from build123d import *

# Parameters (mm, degrees)
SKETCH_2_W               = 120
SKETCH_2_H               = 66
SKETCH_2_W_2             = 112
SKETCH_2_H_2             = 58
EXTRUDE_1_DEPTH          = 2
SKETCH_2_2_W             = 122
SKETCH_2_2_H             = 68
SKETCH_2_2_W_2           = 120
SKETCH_2_2_H_2           = 66
EXTRUDE_1_2_DEPTH        = 4
SKETCH_3_R               = 2
EXTRUDE_2_DEPTH          = 1
SKETCH_4_W               = 10
SKETCH_4_H               = 2
EXTRUDE_3_DEPTH          = 68
EXTRUDE_START            = 12
SKETCH_5_R               = 1.5
EXTRUDE_4_DEPTH          = 1.5
EXTRUDE_START_2          = 16
SKETCH_5_3_R             = 1.5
EXTRUDE_6_DEPTH          = 1.5
FILLET_2_R               = 1
FILLET_2_OF_MIRROR_3_R   = 1
SKETCH_7_W               = 9
SKETCH_7_H               = 5
EXTRUDE_7_DEPTH          = 1
EXTRUDE_8_DEPTH          = 1
EXTRUDE_9_DEPTH          = 1
CUT_EXTRUDE_1_REACH      = 75.022
SKETCH_10_R              = 1.75
MIRROR_6_COPY_1_SKETCH_W = 9
MIRROR_6_COPY_1_SKETCH_H = 5
MIRROR_6_COPY_1_DEPTH    = 1
MIRROR_6_COPY_2_DEPTH    = 1
MIRROR_6_COPY_3_DEPTH    = 1
MIRROR_6_COPY_4_REACH    = 75.022
MIRROR_6_COPY_4_SKETCH_R = 1.75


with BuildPart() as part:
    # 草圖2 → Extrude 1 (new body)
    with BuildSketch(Plane(origin=(0, 0, 0), x_dir=(1, 0, 0), z_dir=(0, 1, 0))):
        Rectangle(SKETCH_2_W, SKETCH_2_H)
        Rectangle(SKETCH_2_W_2, SKETCH_2_H_2, mode=Mode.SUBTRACT)
    extrude(amount=EXTRUDE_1_DEPTH)

    # 草圖2<2> → Extrude 1 2 (add)
    with BuildSketch(Plane(origin=(0, 0, 0), x_dir=(1, 0, 0), z_dir=(0, 1, 0))):
        Rectangle(SKETCH_2_2_W, SKETCH_2_2_H)
        Rectangle(SKETCH_2_2_W_2, SKETCH_2_2_H_2, mode=Mode.SUBTRACT)
    extrude(amount=EXTRUDE_1_2_DEPTH)

    # 草圖3 → 填料-伸長2 (add)
    with BuildSketch(Plane.XY.offset(34)):
        with BuildLine():
            Line((-61, 4), (-57.819768479, 8.731398047))
            ThreePointArc((-57.819768479, 8.731398047), (-54.342718511, 10.496906621), (-51.015153756, 8.463630987))
            Line((-51.015153756, 8.463630987), (-48.5, 4))
            Line((-48.5, 4), (-61, 4))
        make_face()
        with Locations((-54.5, 6.5)):
            Circle(SKETCH_3_R, mode=Mode.SUBTRACT)
    extrude_2 = extrude(amount=-EXTRUDE_2_DEPTH)

    # 鏡射1: 填料-伸長2 across plane
    add(extrude_2.mirror(Plane.XY))

    # 草圖4 → 填料-伸長3 (add)
    with BuildSketch(Plane.XY.offset(34)):
        with Locations((11, 1)):
            Rectangle(SKETCH_4_W, SKETCH_4_H)
    extrude(amount=-EXTRUDE_3_DEPTH)

    # 草圖5 → 填料-伸長4 (add)
    with BuildSketch(Plane.XY.offset(EXTRUDE_START)):
        with BuildLine():
            Line((8.5, 4.5), (8.5, 2))
            Line((8.5, 2), (13.5, 2))
            Line((13.5, 2), (13.5, 4.5))
            ThreePointArc((13.5, 4.5), (11, 7), (8.5, 4.5))
        make_face()
        with Locations((11, 4.5)):
            Circle(SKETCH_5_R, mode=Mode.SUBTRACT)
    extrude_4 = extrude(amount=EXTRUDE_4_DEPTH)

    # 草圖5<3> → 填料-伸長6 (add)
    with BuildSketch(Plane.XY.offset(EXTRUDE_START_2)):
        with BuildLine():
            Line((8.5, 4.5), (8.5, 2))
            Line((8.5, 2), (13.5, 2))
            Line((13.5, 2), (13.5, 4.5))
            ThreePointArc((13.5, 4.5), (11, 7), (8.5, 4.5))
        make_face()
        with Locations((11, 4.5)):
            Circle(SKETCH_5_3_R, mode=Mode.SUBTRACT)
    extrude_6 = extrude(amount=EXTRUDE_6_DEPTH)

    # 圓角2
    fillet_2_edges = [part.edges().sort_by_distance(p)[0] for p in [
        (11, 2, 13.5),
        (11, 2, 12),
        (8.5, 2, 12.75),
        (13.5, 2, 12.75),
        (11, 2, 17.5),
        (11, 2, 16),
        (8.5, 2, 16.75),
        (13.5, 2, 16.75),
    ]]
    fillet(fillet_2_edges, radius=FILLET_2_R - 0.0001)  # a hair under: the kernel refuses the full size

    # 鏡射3: 填料-伸長4, 填料-伸長6 across plane
    add(extrude_4.mirror(Plane.XY))
    add(extrude_6.mirror(Plane.XY))

    # 圓角2 of 鏡射3
    fillet_2_of_mirror_3_edges = [part.edges().sort_by_distance(p)[0] for p in [
        (11, 2, -13.5),
        (11, 2, -12),
        (8.5, 2, -12.75),
        (13.5, 2, -12.75),
        (11, 2, -17.5),
        (11, 2, -16),
        (8.5, 2, -16.75),
        (13.5, 2, -16.75),
    ]]
    fillet(fillet_2_of_mirror_3_edges, radius=FILLET_2_OF_MIRROR_3_R - 0.0001)  # a hair under: the kernel refuses the full size

    # 草圖7 → 填料-伸長7 (add)
    with BuildSketch(Plane.XZ):
        with Locations((38.5, 36.5)):
            Rectangle(SKETCH_7_W, SKETCH_7_H)
    extrude_7 = extrude(amount=-EXTRUDE_7_DEPTH)

    # 草圖8 → 填料-伸長8 (add)
    with BuildSketch(Plane(origin=(43, 0, 0), x_dir=(0, 0, -1), z_dir=(1, 0, 0))):
        Polygon((-39, 1), (-34, 4), (-34, 1), align=None)
    extrude_8 = extrude(amount=-EXTRUDE_8_DEPTH)

    # 草圖9 → 填料-伸長9 (add)
    with BuildSketch(Plane.ZY.offset(-34)):
        Polygon((39, 1), (34, 4), (34, 1), align=None)
    extrude_9 = extrude(amount=-EXTRUDE_9_DEPTH)

    # 草圖10 → 除料-伸長1 (cut, up to next)
    with BuildSketch(Plane(origin=(0, 1, 0), x_dir=(1, 0, 0), z_dir=(0, 1, 0)), mode=Mode.PRIVATE) as cut_extrude_1_sk1:
        with Locations(Location((38.5, -36.5, 0), (0, 0, 270))):
            Circle(SKETCH_10_R)
    cut_extrude_1_tool1 = extrude(cut_extrude_1_sk1.sketch, amount=-CUT_EXTRUDE_1_REACH, mode=Mode.PRIVATE) & part.part
    cut_extrude_1 = cut_extrude_1_tool1.solids().sort_by_distance((38.5, 1, 36.5))[0]
    add(cut_extrude_1, mode=Mode.SUBTRACT)

    # 鏡射5: 填料-伸長7, 填料-伸長8, 填料-伸長9, 除料-伸長1 across plane
    add(extrude_7.mirror(Plane.XY))
    add(extrude_8.mirror(Plane.XY))
    add(extrude_9.mirror(Plane.XY))
    add(cut_extrude_1.mirror(Plane.XY), mode=Mode.SUBTRACT)

    # 鏡射6: 填料-伸長7, 填料-伸長8, 填料-伸長9, 除料-伸長1 across plane
    add(extrude_7.mirror(Plane(origin=(0, 0, 0), x_dir=(0, 0, 1), z_dir=(1, 0, 0))))
    add(extrude_8.mirror(Plane(origin=(0, 0, 0), x_dir=(0, 0, 1), z_dir=(1, 0, 0))))
    add(extrude_9.mirror(Plane(origin=(0, 0, 0), x_dir=(0, 0, 1), z_dir=(1, 0, 0))))
    add(cut_extrude_1.mirror(Plane(origin=(0, 0, 0), x_dir=(0, 0, 1), z_dir=(1, 0, 0))), mode=Mode.SUBTRACT)

    # 鏡射6 copy 1 sketch → 鏡射6 copy 1 (add)
    with BuildSketch(Plane(origin=(0, 0, 0), x_dir=(-1, 0, 0), z_dir=(0, -1, 0))):
        with Locations((38.5, 36.5)):
            Rectangle(MIRROR_6_COPY_1_SKETCH_W, MIRROR_6_COPY_1_SKETCH_H)
    extrude(amount=-MIRROR_6_COPY_1_DEPTH)

    # 鏡射6 copy 2 sketch → 鏡射6 copy 2 (add)
    with BuildSketch(Plane.ZY.offset(43)):
        Polygon((-39, 1), (-34, 4), (-34, 1), align=None)
    extrude(amount=-MIRROR_6_COPY_2_DEPTH)

    # 鏡射6 copy 3 sketch → 鏡射6 copy 3 (add)
    with BuildSketch(Plane(origin=(-34, 0, 0), x_dir=(0, 0, -1), z_dir=(1, 0, 0))):
        Polygon((39, 1), (34, 4), (34, 1), align=None)
    extrude(amount=-MIRROR_6_COPY_3_DEPTH)

    # 鏡射6 copy 4 sketch → 鏡射6 copy 4 (cut, up to next)
    with BuildSketch(Plane(origin=(0, 1, 0), x_dir=(-1, 0, 0), z_dir=(0, 1, 0)), mode=Mode.PRIVATE) as mirror_6_copy_4_sk1:
        with Locations(Location((38.5, -36.5, 0), (0, 0, 270))):
            Circle(MIRROR_6_COPY_4_SKETCH_R)
    mirror_6_copy_4_tool1 = extrude(mirror_6_copy_4_sk1.sketch, amount=-MIRROR_6_COPY_4_REACH, mode=Mode.PRIVATE) & part.part
    add(mirror_6_copy_4_tool1.solids().sort_by_distance((-38.5, 1, -36.5))[0], mode=Mode.SUBTRACT)


solid = part.part
Read the model definition and answer for the solid it produces. Units are mm, in the model's axes. A direction names the side the tool comes from. Round coordinates to 2 decimals unless told otherwise and drop trailing zeros. Loops run counter-clockwise (first coordinate to the right, second up) from the corner with the lowest first, then second, coordinate; pieces in that order, holes last. Notation, with made-up numbers: (44.5, 29.5) - (86.5, 29.5) arc R3 cw to (86.5, 33.5) - close; hole circle Ø3 at (-31, 73.5). An arc over 180 degrees is marked (long way). One line per question, with ' | ' between items. Start each with the question number.
Q1. Section B-B on x = -15.5 is taken. Give the vertices of the cut face in (y, z).
Q2. Flat-ended cylindrical pins translate along their axes: pin 1 (2 mm diameter, centred on y = 2, z = 37.5, fed in from -X); pin 2 (3 mm diameter, centred on x = 11, y = 4, fed in from +Z); pin 3 (5.5 mm diameter, centred on x = -37.5, z = -37, fed in from +Y); pin 4 (6 mm diameter, centred on y = 5, z = 21.5, fed in from -X). Find the tip coordinate at first contact, or state that the pin passes through.
Q3. Section A-A on z = -8.5 is taken. Give the vertices of the cut face in (x, y).
Q4. Section C-C on x = -38.5 is taken. Give the vertices of the cut face in (y, z).
Q5. Section D-D on z = 36.5 is taken. Give the vertices of the cut face in (x, y), plus the area to 3 significant figures.
Q6. Find the intervals of material crossed by L1, parallel to X at y = 0.6, z = 36.5; L2, parallel to Z at x = -38.5, y = 0.65; L3, parallel to Z at x = 9.5, y = 5, in increasing order.
Q7. For faces 4 (the flat face through (-39, 3, 34)), 5 (the flat face through (52, 2, -34)), 6 (the flat face through (35, 2, -35)), 7 (the cylindrical face through (9.5, 4.57, 12.74)), 8 (the flat face through (-54, 4, 34)), determine the directions among +Z, -Z, +X, -X, +Y, -Y from which every point of the face is accessible in a straight line to the end or side of a thin tool.
Q8. For a pull along Y with two mould halves and no side action, classify faces 1 (the flat face through (12, 6, 12)), 2 (the cylindrical face through (9.5, 4.57, 16.74)), 3 (the flat face through (34.5, 2.5, -36.5)) as +Y half, -Y half, draft (parallel to the pull), parting line (faces both ways), or undercut.
Established:
1) outline: (0, -34) - (4, -34) - (4, -33) - (2, -33) - (2, -29) - (0, -29) - close; (0, 29) - (2, 29) - (2, 33) - (4, 33) - (4, 34) - (0, 34) - close
2) pin 1: x = -43 | pin 2: z = 34 | pin 3: y = 2.89 | pin 4: x = -61
3) outline: (-61, 0) - (-56, 0) - (-56, 2) - (-60, 2) - (-60, 4) - (-61, 4) - close; (6, 0) - (16, 0) - (16, 2) - (6, 2) - close; (56, 0) - (61, 0) - (61, 4) - (60, 4) - (60, 2) - (56, 2) - close
4) outline: (0, -39) - (1, -39) - (1, -38.25) - (0, -38.25) - close; (0, -34.75) - (1, -34.75) - (1, -34) - (4, -34) - (4, -33) - (2, -33) - (2, -29) - (0, -29) - close; (0, 29) - (2, 29) - (2, 33) - (4, 33) - (4, 34) - (1, 34) - (1, 34.75) - (0, 34.75) - close; (0, 38.25) - (1, 38.25) - (1, 39) - (0, 39) - close
5) outline: (-43, 0) - (-40.25, 0) - (-40.25, 1) - (-42, 1) - (-42, 2.5) - (-43, 2.5) - close; (-36.75, 0) - (-34, 0) - (-34, 2.5) - (-35, 2.5) - (-35, 1) - (-36.75, 1) - close; (34, 0) - (36.75, 0) - (36.75, 1) - (35, 1) - (35, 2.5) - (34, 2.5) - close; (40.25, 0) - (43, 0) - (43, 2.5) - (42, 2.5) - (42, 1) - (40.25, 1) - close | area: 17.0 mm²
6) L1: -43 to -40.25, -36.75 to -34, 34 to 36.75, 40.25 to 43 | L2: -39 to -38.25, -34.75 to -29, 29 to 34.75, 38.25 to 39 | L3: -17.5 to -16, -13.5 to -12, 12 to 13.5, 16 to 17.5
7) face 4: +Z, +Y | face 5: -Z, +X, +Y, -Y | face 6: -Z, +Y | face 7: none | face 8: +Z, -X, +Y, -Y
8) face 1: draft | face 2: undercut | face 3: +Y half
